Here's the drawing with two shaded views (mm, measured from the low corner). I have some questions. Give positions to 0.01 mm unless a question says otherwise; leave off trailing zeros. Loops run counter-clockwise (first coordinate to the right, second up) from the corner with the lowest first, then second, coordinate; pieces in that order, holes last. Notation, with made-up numbers: (71.25, -31) -> (90.25, -31) arc R21 cw to (90.25, -11) -> close; hole circle Ø4 at (53, -11). An arc over 180 degrees is marked (long way). Put each result on its own line as item: value.
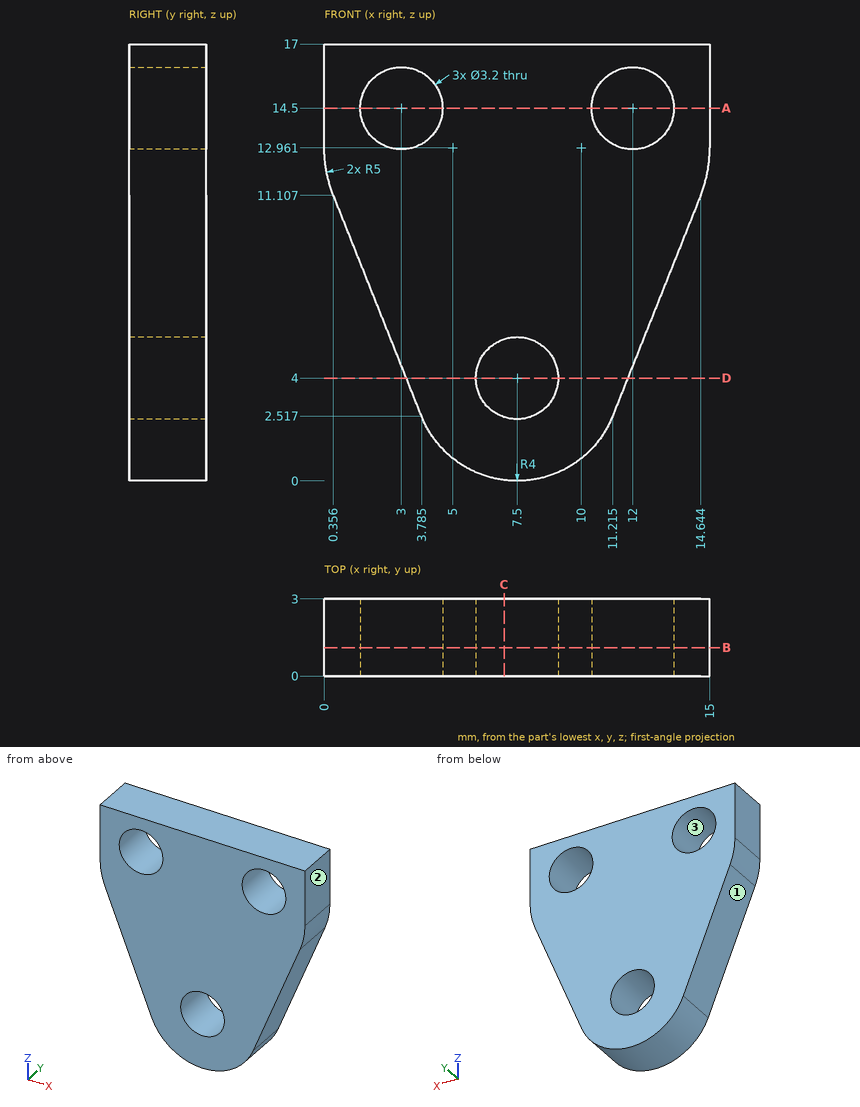
1. If we section it at B-B (y = 1.1): List the corners of the cut face in (x, z) for me (1 decimal), then the cut area to 3 significant figures.
Recorded:
outline: (0, 13) arc R5 ccw to (0.4, 11.1) -> (3.8, 2.5) arc R4 ccw to (11.2, 2.5) -> (14.6, 11.1) arc R5 ccw to (15, 13) -> (15, 17) -> (0, 17) -> close; hole circle Ø3.2 at (3, 14.5); hole circle Ø3.2 at (7.5, 4); hole circle Ø3.2 at (12, 14.5)
area: 171 mm^2
2. If we section it at C-C (x = 7): List the corners of the cut face in (y, z) for me.
Recorded:
outline: (0, 0.03) -> (3, 0.03) -> (3, 2.48) -> (0, 2.48) -> close; (0, 5.52) -> (3, 5.52) -> (3, 17) -> (0, 17) -> close
3. I'm going to push a flat-ended pin straight in: pin 1 (1.9 mm diameter, centred on x = 12, z = 14.5, fed in from +Y). Where does the tip first touch, or does it pass through?
Recorded:
pin 1: passes through
4. I need wall thicknesses on line 1 (X direction, y = 2.4, z = 14.5); line 2 (Z direction, x = 10.75, y = 2.85) (1 decimal); line 3 (X direction, y = 1.35, z = 4). Which ranges of each line are inside material? Lowest first, please.
Recorded:
line 1: x = 0 to 1.4, 4.6 to 10.4, 13.6 to 15
line 2: z = 1.7 to 13.5, 15.5 to 17
line 3: x = 3.19 to 5.9, 9.1 to 11.81
5. If we section it at D-D (z = 4): List the corners of the cut face in (x, y) for me.
Recorded:
outline: (3.19, 0) -> (5.9, 0) -> (5.9, 3) -> (3.19, 3) -> close; (9.1, 0) -> (11.81, 0) -> (11.81, 3) -> (9.1, 3) -> close
6. Thinking about a two-plate mould opening in Z: for the marked faces 1, 2 and 3, which applies, pulls with the +Z half, pulls with the -Z half, needs draft (parallel to the pull), parting line crosses it, or undercut?
Recorded:
face 1: pulls with the -Z half
face 2: needs draft
face 3: undercut
7. If we section it at A-A (z = 14.5): List the corners of the cut face in (x, y) for me, then the cut area to 3 significant figures.
Recorded:
outline: (0, 0) -> (1.4, 0) -> (1.4, 3) -> (0, 3) -> close; (4.6, 0) -> (10.4, 0) -> (10.4, 3) -> (4.6, 3) -> close; (13.6, 0) -> (15, 0) -> (15, 3) -> (13.6, 3) -> close
area: 25.8 mm^2
